Input: part model. Units: mm. Frame: model coordinates. Face numbers are marked on the shaded views. A direction names the side the tool comes from. Round coordinates to 2 decimals unless told otherwise and drop trailing zeros. Loops run counter-clockwise (first coordinate to the right, second up) from the corner with the lowest first, then second, coordinate; pieces in that order, holes last.
(1) Line query: line 1 (Z direction, x = 8.5, y = 16.5); line 2 (X direction, y = 25.5, z = -29.5); line 3 (Z direction, x = 18.25, y = 15.5). Output: solid intervals per line, ascending.
(2) Draft query along Z for the marked faces 4, 5 and 6. Return one class per face: released by +Z, released by -Z, zero draft, split by the parting line, or undercut.
(3) Cut plane A-A, the plane x = 10. Output: boundary loops of the cut face in (y, z).
(4) First-contact query: pin 1 Ø4.5 at (x, z) = (10, -83.15) entering from +Y; pin 2 Ø4 at (x, y) = (9, 27.5) entering from +Z; pin 3 Ø8 at (x, y) = (9, 12) entering from -Z. Flat tips, straight axial feed; report the tip coordinate or a pass-through.
(5) Cut plane D-D, the plane x = 2. Output: boundary loops of the cut face in (y, z).
(6) Cut plane C-C, the plane y = 14. Output: boundary loops of the cut face in (x, z).
(7) Cut plane B-B, the plane z = -6.25. Output: boundary loops of the cut face in (x, y).
(8) Access query for the marked faces 1, 2 and 3. Directions: +Z, -Z, +X, -X, +Y, -Y. A direction counts if a zero-diameter tool reaches every point of the face in a straight line with its end or side. Return the directions, or none.
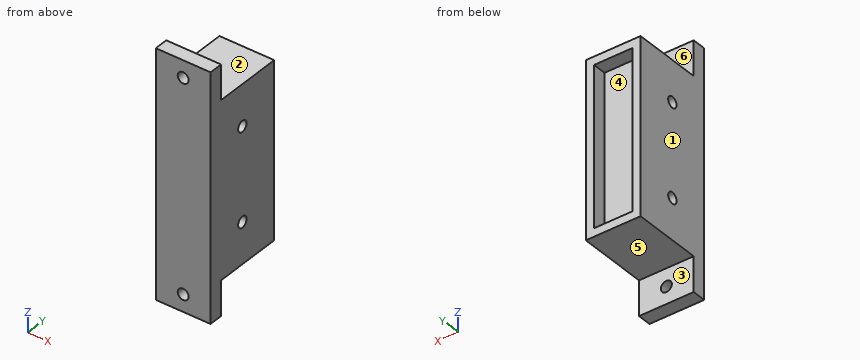
from build123d import *

# Parameters (mm, degrees)
BOSS_EXTRUDE1_DEPTH     = 20
SKETCH4_W               = 14
SKETCH4_H               = 58
CUT_EXTRUDE1_DEPTH      = 5
SKETCH5_R               = 2
CUT_EXTRUDE2_DEPTH      = 5
CUT_EXTRUDE3_DEPTH      = 97.522121817
CUT_EXTRUDE3_DEPTH_BACK = 5
SKETCH6_R               = 2


with BuildPart() as part:
    # Sketch1 → Boss-Extrude1 (new body)
    with BuildSketch(Plane(origin=(0, 0, 0), x_dir=(0, 0, -1), z_dir=(1, 0, 0))):
        Polygon((0, 0), (0, 5), (12.7, 5), (12.7, 30.4), (76.7, 30.4), (76.7, 5), (89.4, 5), (89.4, 0), align=None)
    extrude(amount=BOSS_EXTRUDE1_DEPTH)

    # Sketch4 → Cut-Extrude1 (cut)
    with BuildSketch(Plane(origin=(0, 30.4, 0), x_dir=(1, 0, 0), z_dir=(0, 1, 0))):
        with Locations((9.986416009, 44.7)):
            Rectangle(SKETCH4_W, SKETCH4_H)
    extrude(amount=-CUT_EXTRUDE1_DEPTH, mode=Mode.SUBTRACT)

    # Sketch5 → Cut-Extrude2 (cut)
    with BuildSketch(Plane(origin=(0, 5, 0), x_dir=(1, 0, 0), z_dir=(0, 1, 0))):
        with Locations(Location((10, 83.15, 0), (0, 0, 270))):
            Circle(SKETCH5_R)
        with Locations(Location((10, 6.25, 0), (0, 0, 270))):
            Circle(SKETCH5_R)
    extrude(amount=-CUT_EXTRUDE2_DEPTH, mode=Mode.SUBTRACT)

    # Sketch6 → Cut-Extrude3 (cut, two sides: drawn at the far end of the back side and taken through both)
    with BuildSketch(Plane(origin=(0, 0, 0), x_dir=(0, 0, -1), z_dir=(1, 0, 0)).offset(-CUT_EXTRUDE3_DEPTH_BACK)):
        with Locations(Location((27.7, 15.2, 0), (0, 0, 180))):
            Circle(SKETCH6_R)
        with Locations(Location((61.7, 15.2, 0), (0, 0, 180))):
            Circle(SKETCH6_R)
    extrude(amount=CUT_EXTRUDE3_DEPTH + CUT_EXTRUDE3_DEPTH_BACK, mode=Mode.SUBTRACT)


solid = part.part
Reported:
1. line 1: z = -76.7 to -63.22, -60.18 to -29.22, -26.18 to -12.7
1. line 2: x = 0 to 2.99, 16.99 to 20
1. line 3: z = -76.7 to -63.68, -59.72 to -29.68, -25.72 to -12.7
2. face 4: undercut
2. face 5: released by -Z
2. face 6: zero draft
3. outline: (0, -89.4) - (5, -89.4) - (5, -85.15) - (0, -85.15) - close; (0, -81.15) - (5, -81.15) - (5, -76.7) - (30.4, -76.7) - (30.4, -73.7) - (25.4, -73.7) - (25.4, -15.7) - (30.4, -15.7) - (30.4, -12.7) - (5, -12.7) - (5, -8.25) - (0, -8.25) - close; (0, -4.25) - (5, -4.25) - (5, 0) - (0, 0) - close; hole circle Ø4 at (15.2, -61.7); hole circle Ø4 at (15.2, -27.7)
4. pin 1: stops at y = 5
4. pin 2: stops at z = -12.7
4. pin 3: stops at z = -76.7
5. outline: (0, -89.4) - (5, -89.4) - (5, -76.7) - (30.4, -76.7) - (30.4, -12.7) - (5, -12.7) - (5, 0) - (0, 0) - close; hole circle Ø4 at (15.2, -61.7); hole circle Ø4 at (15.2, -27.7)
6. outline: (0, -76.7) - (20, -76.7) - (20, -63.3) - (0, -63.3) - close; (0, -60.1) - (20, -60.1) - (20, -29.3) - (0, -29.3) - close; (0, -26.1) - (20, -26.1) - (20, -12.7) - (0, -12.7) - close
7. outline: (0, 0) - (8, 0) - (8, 5) - (0, 5) - close; (12, 0) - (20, 0) - (20, 5) - (12, 5) - close
8. face 1: +Z, -Z, -X, +Y, -Y
8. face 2: +Z, +X, -X, +Y
8. face 3: -Z, +X, -X, +Y
